```python
from build123d import *

# Parameters (mm, degrees)
BOSS_EXTRUDE2_DEPTH  = 3.175
BOSS_EXTRUDE3_DEPTH  = 3.175
BOSS_EXTRUDE6_DEPTH  = 3.175
SKETCH8_W            = 70.49262
SKETCH8_H            = 3.175
BOSS_EXTRUDE7_DEPTH  = 3.175
M4_CLEARANCE_HOLE2_D = 4.8


with BuildPart() as part:
    # Sketch1 → Boss-Extrude2 (new body)
    with BuildSketch(Plane.XY):
        Polygon((129.013076168, 254.245404572), (-18.685383832, 254.245404572), (-18.685383832, 157.666984572), (92.088461168, 157.666984572), (92.088461168, 154.491984572), (-18.685383832, 154.491984572), (-18.685383832, 57.913564572), (92.088461168, 57.913564572), (92.088461168, 54.738564572), (-18.685383832, 54.738564572), (-18.685383832, -41.839855428), (92.088461168, -41.839855428), (92.088461168, -45.014855428), (-18.685383832, -45.014855428), (-18.685383832, -141.593275428), (92.088461168, -141.593275428), (92.088461168, -144.768275428), (-18.685383832, -144.768275428), (-18.685383832, -241.346695428), (129.013076168, -241.346695428), align=None)
    extrude(amount=BOSS_EXTRUDE2_DEPTH)

    # Sketch2 → Boss-Extrude3 (add, through all)
    with BuildSketch(Plane.XY.offset(3.175)):
        Polygon((129.013076168, 254.245404572), (129.013076168, -241.346695428), (153.407236168, -241.346695428), (153.407236168, -227.262720585), (153.407236168, -187.892720585), (153.407236168, -143.180775428), (153.407236168, 240.16142973), (153.407236168, 254.245404572), align=None)
    extrude(amount=-BOSS_EXTRUDE3_DEPTH)

    # Sketch7 → Boss-Extrude6 (add, through all)
    with BuildSketch(Plane.XY.offset(3.175)):
        Polygon((153.22938521, -141.593275428), (153.407236168, -64.827061449), (266.437236168, -64.827061449), (266.437236168, -141.593275428), align=None)
    extrude(amount=-BOSS_EXTRUDE6_DEPTH)

    # Sketch8 → Boss-Extrude7 (add, through all)
    with BuildSketch(Plane.XY.offset(3.175)):
        with Locations((16.560926168, 255.832904572)):
            Rectangle(SKETCH8_W, SKETCH8_H)
        with Locations((16.560926168, -242.934195428)):
            Rectangle(SKETCH8_W, SKETCH8_H)
    extrude(amount=-BOSS_EXTRUDE7_DEPTH)

    # M4 Clearance Hole2 (through all)
    with Locations(Plane.XY.offset(3.175)):
        with Locations((143.247236168, 244.013297791), (143.247236168, 171.121259486), (143.247236168, 98.229221182), (143.247236168, 25.337182877), (143.247236168, -47.554855428), (170.679236168, -74.986855428), (210.711682777, -74.986855428), (250.744129387, -74.986855428), (256.277236168, -80.519962209), (256.277236168, -106.747508818), (256.277236168, -132.975055428), (143.247236168, -160.673755428), (143.247236168, -195.894172037), (143.247236168, -231.114588646)):
            Hole(M4_CLEARANCE_HOLE2_D / 2)


solid = part.part
```
Input: part model. Units: mm. Frame: model coordinates. Round coordinates to 2 decimals unless told otherwise and drop trailing zeros. Order: outer loops, then holes, each group sorted by start corner. A loop starts at its lowest first (then second) coordinate and runs counter-clockwise, first axis right, second up. Notation, with made-up numbers: (24.25, 46) - (30.25, 46) arc R37 cw to (30.25, 82) - close; hole circle Ø5 at (86.25, 52.5). An arc over 180 degrees is marked (long way). Answer in a Markdown table with one row per item.
Item 1: Section query D-D (z = 2.4). Give the number of separate pieces and of enclosed holes in the cut face, then the cut area to 3 significant figures.
Model answer:
| item | result |
|---|---|
| separate pieces | 1 |
| enclosed holes | 14 |
| area | 92,800 mm² |
Item 2: Pin query (flat end, axial travel): pin 1 (1.6 mm diameter, centred on y = -143, z = 1, fed in from -X). Return the tip coordinate at first contact, or that it passes through.
Model answer:
| item | result |
|---|---|
| pin 1 | stops at x = 92.09 |
Item 3: Section query B-B (x = 79.5). Return the cut outline in (y, z) (3 decimals).
Model answer:
| item | result |
|---|---|
| outline | (-241.347, 0) - (-144.768, 0) - (-144.768, 3.175) - (-241.347, 3.175) - close; (-141.593, 0) - (-45.015, 0) - (-45.015, 3.175) - (-141.593, 3.175) - close; (-41.84, 0) - (54.739, 0) - (54.739, 3.175) - (-41.84, 3.175) - close; (57.914, 0) - (154.492, 0) - (154.492, 3.175) - (57.914, 3.175) - close; (157.667, 0) - (254.245, 0) - (254.245, 3.175) - (157.667, 3.175) - close |
Item 4: Section query A-A (x = 7). Return the cut outline in (y, z) (3 decimals).
Model answer:
| item | result |
|---|---|
| outline | (-244.522, 0) - (-144.768, 0) - (-144.768, 3.175) - (-244.522, 3.175) - close; (-141.593, 0) - (-45.015, 0) - (-45.015, 3.175) - (-141.593, 3.175) - close; (-41.84, 0) - (54.739, 0) - (54.739, 3.175) - (-41.84, 3.175) - close; (57.914, 0) - (154.492, 0) - (154.492, 3.175) - (57.914, 3.175) - close; (157.667, 0) - (257.42, 0) - (257.42, 3.175) - (157.667, 3.175) - close |
Item 5: Line query: line 1 (Y direction, x = 12, z = 2.6); line 2 (Y direction, x = 60, z = 1.05); line 3 (X direction, y = -75.5, z = 3). Output: solid intervals per line, ascending.
Model answer:
| item | result |
|---|---|
| line 1 | y = -244.52 to -144.77, -141.59 to -45.01, -41.84 to 54.74, 57.91 to 154.49, 157.67 to 257.42 |
| line 2 | y = -241.35 to -144.77, -141.59 to -45.01, -41.84 to 54.74, 57.91 to 154.49, 157.67 to 254.25 |
| line 3 | x = -18.69 to 168.33, 173.02 to 208.37, 213.06 to 248.4, 253.09 to 266.44 |
Item 6: Section query C-C (y = -60). Return the cut outline in (x, z) (3 decimals).
Model answer:
| item | result |
|---|---|
| outline | (-18.685, 0) - (153.407, 0) - (153.407, 3.175) - (-18.685, 3.175) - close |
